from build123d import *

# Parameters (mm, degrees)
SKETCH_W     = 52.1
SKETCH_H     = 29.9
SKETCH_W_2   = 6.2
SKETCH_H_2   = 15.4
PAD_DEPTH    = 7
SKETCH001_W  = 50.1
SKETCH001_H  = 27.9
POCKET_DEPTH = 6


with BuildPart() as part:
    # Sketch → Pad (new body)
    with BuildSketch(Plane.XY):
        Rectangle(SKETCH_W, SKETCH_H)
        Rectangle(SKETCH_W_2, SKETCH_H_2, mode=Mode.SUBTRACT)
    extrude(amount=PAD_DEPTH)

    # Sketch001 (on Face9 of Pad) → Pocket (cut)
    with BuildSketch(Plane(origin=(0, 0, 0), x_dir=(1, 0, 0), z_dir=(0, 0, -1))):
        Rectangle(SKETCH001_W, SKETCH001_H)
    extrude(amount=-POCKET_DEPTH, mode=Mode.SUBTRACT)


solid = part.part
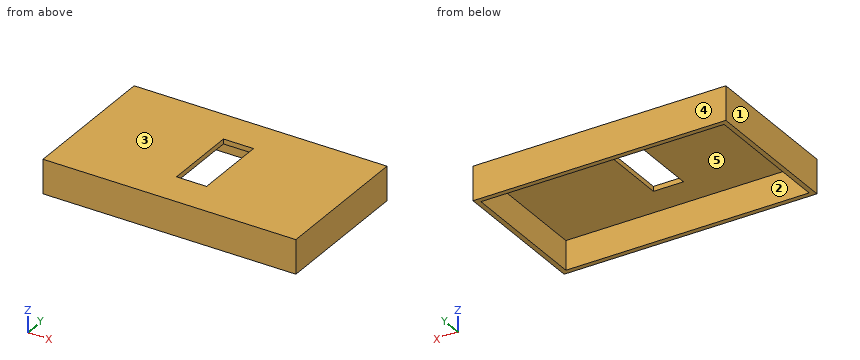
Work out the finished part from the listing and answer in its coordinate system (mm). Face numbers are marked on the shaded views. A direction names the side the tool comes from. Coordinates: 2 decimals unless noted, no trailing zeros. Write each loop counter-clockwise with the first axis right and the second up, starting at its lowest first coordinate (ties: lowest second). Pieces come first, ordered by that corner, then holes. Notation, with made-up numbers: (82, 76.25) - (128, 76.25) arc R18 cw to (128, 93.25) - close; hole circle Ø5 at (14.5, -27.5). An arc over 180 degrees is marked (long way). One line per question, with ' | ' between items.
1) Find section D-D, the plane x = 8.5. Determine the outline of the cut face in (y, z), and give its area (3 significant figures).
Checks:
outline: (-14.95, 0) - (-13.95, 0) - (-13.95, 6) - (13.95, 6) - (13.95, 0) - (14.95, 0) - (14.95, 7) - (-14.95, 7) - close | area: 41.9 mm2
2) Find section A-A, the plane y = -0.75. Determine the outline of the cut face in (x, z).
Checks:
outline: (-26.05, 0) - (-25.05, 0) - (-25.05, 6) - (-3.1, 6) - (-3.1, 7) - (-26.05, 7) - close; (3.1, 6) - (25.05, 6) - (25.05, 0) - (26.05, 0) - (26.05, 7) - (3.1, 7) - close
3) Find section B-B, the plane z = 4.5. Determine the outline of the cut face in (x, y).
Checks:
outline: (-26.05, -14.95) - (26.05, -14.95) - (26.05, 14.95) - (-26.05, 14.95) - close; hole (-25.05, -13.95) - (25.05, -13.95) - (25.05, 13.95) - (-25.05, 13.95) - close
4) The mould has two halves that part along X. Classify the marked faces 1, 2 and 3: +X half, -X half, draft (parallel to the pull), parting line (faces both ways), or undercut.
Checks:
face 1: -X half | face 2: undercut | face 3: draft
5) For the marked faces 4 and 5, determine the directions among +Z, -Z, +X, -X, +Y, -Y from which every point of the face is accessible in a straight line to the end or side of a thin tool.
Checks:
face 4: +Z, -Z, +X, -X, +Y | face 5: -Z
6) Find section C-C, the plane y = 10.5. Determine the outline of the cut face in (x, z).
Checks:
outline: (-26.05, 0) - (-25.05, 0) - (-25.05, 6) - (25.05, 6) - (25.05, 0) - (26.05, 0) - (26.05, 7) - (-26.05, 7) - close
7) A flat-ended cylindrical pin translates along its axis: P1, Ø1.5, axis at x = -3, y = 8.5, coming from the -Z side. Find the tip coordinate at first contact, or state that the pin passes through.
Checks:
P1: z = 6
8) Consider probe 1 along X at (y, z) = (-12.25, 3.5); probe 2 along Y at (x, z) = (12, 4); probe 3 along X at (y, z) = (2.5, 6.75). Determine where each line is inside the solid, lowest interval first. Write a range as [from, to].
Checks:
probe 1: [-26.05, -25.05], [25.05, 26.05] | probe 2: [-14.95, -13.95], [13.95, 14.95] | probe 3: [-26.05, -3.1], [3.1, 26.05]
